The listing builds one solid part. Answer for the finished solid, in the listing's coordinates (mm). A direction names the side the tool comes from. Coordinates: 2 decimals unless noted, no trailing zeros. Order: outer loops, then holes, each group sorted by start corner. A loop starts at its lowest first (then second) coordinate and runs counter-clockwise, first axis right, second up. Notation, with made-up numbers: (-35, 4) -> (19, 4) arc R22 ccw to (19, 25) -> close; hole circle Ø3 at (23.5, 88.25). An arc over 180 degrees is marked (long way). Write each question's results on one line, items separated by ' | '. Start each with the question number.
(1) The part is cut by section B-B, the plane x = 61.5. Give the vertices of the cut face in (y, z).
(2) Straight lines are drawn through the part: L1, parallel to X at y = 6.75, z = -51; L2, parallel to X at y = 14.5, z = -8.5; L3, parallel to Z at x = 65, y = 19.75. For each, find the intervals that lie inside material, in ascending order.
(3) The part is cut by section C-C, the plane y = 10. Give the vertices of the cut face in (x, z), then the cut area to 3 significant figures.
(4) The part is cut by section D-D, the plane x = 87.5. Give the vertices of the cut face in (y, z), then the cut area to 3 significant figures.
(5) The part is cut by section A-A, the plane y = 21.5. Give the vertices of the cut face in (x, z), then the cut area to 3 significant figures.
(6) Determine the mould class of faces 4 (the face through (100, 12, -49)), 5 (the face through (50, 25, -10)), 6 (the face through (72, 14, -10)) for opening direction X: +X half, -X half, draft (parallel to the pull), parting line (faces both ways), or undercut.
(7) Given pin 1 (1.9 mm diameter, centred on x = 82, z = -57, fed in from +Y); pin 2 (3 mm diameter, centred on x = 70.5, z = -5.5, fed in from +Y); pin 3 (4 mm diameter, centred on x = 35, z = -68, fed in from +Y), each flat-ended and moving along its own axis, determine where each tip first touches the part or whether it passes through.
(8) A tool of negligible diameter and unlimited length cuts with its end or side. For faces 1 (the face through (86, 2, -72)), 2 (the face through (49, 18, -2.4)), 3 (the face through (49, 12, -100)), from which of +Z, -Z, +X, -X, +Y, -Y can it reach the whole face along a straight path? Write none if from no direction.
```python
from build123d import *

# Parameters (mm, degrees)
CROQUIS1_W              = 100
CROQUIS1_H              = 100
PLACABASE_DEPTH         = 3
CROQUIS2_W              = 100
CROQUIS2_H              = 100
CROQUIS2_W_2            = 95.2
CROQUIS2_H_2            = 95.2
PAREDES_DEPTH           = 21
CROQUIS4_W              = 26.4
CROQUIS4_H              = 10.4
ALOJAMIENTOSMOTOR_DEPTH = 12.4
CROQUIS6_W              = 2.4
CROQUIS6_H              = 95.2
NERVIOSRIGIDEZ_DEPTH    = 9
CROQUIS7_W              = 95.2
CROQUIS7_H              = 6
BLOQUECUNA_DEPTH        = 10
CROQUIS8_W              = 44
CROQUIS8_H              = 4
TORRESENSORES_DEPTH     = 22


with BuildPart() as part:
    # Croquis1 → PlacaBase (new body)
    with BuildSketch(Plane(origin=(0, 0, 0), x_dir=(1, 0, 0), z_dir=(0, 1, 0))):
        with Locations((50, 50)):
            Rectangle(CROQUIS1_W, CROQUIS1_H)
    extrude(amount=PLACABASE_DEPTH)

    # Croquis2 → Paredes (add)
    with BuildSketch(Plane(origin=(0, 3, 0), x_dir=(1, 0, 0), z_dir=(0, 1, 0))):
        with Locations((50, 50)):
            Rectangle(CROQUIS2_W, CROQUIS2_H)
        with Locations((50, 50)):
            Rectangle(CROQUIS2_W_2, CROQUIS2_H_2, mode=Mode.SUBTRACT)
    extrude(amount=PAREDES_DEPTH)

    # Croquis4 → AlojamientosMotor (cut)
    with BuildSketch(Plane(origin=(0, 7.3, 0), x_dir=(1, 0, 0), z_dir=(0, 1, 0))):
        with Locations((27.2, 72)):
            Rectangle(CROQUIS4_W, CROQUIS4_H)
        with Locations((72.8, 72)):
            Rectangle(CROQUIS4_W, CROQUIS4_H)
    extrude(amount=-ALOJAMIENTOSMOTOR_DEPTH, mode=Mode.SUBTRACT)

    # Croquis6 → NerviosRigidez (add)
    with BuildSketch(Plane(origin=(0, 3, 0), x_dir=(1, 0, 0), z_dir=(0, 1, 0))):
        with Locations((18.2, 50)):
            Rectangle(CROQUIS6_W, CROQUIS6_H)
        with Locations((81.8, 50)):
            Rectangle(CROQUIS6_W, CROQUIS6_H)
    extrude(amount=NERVIOSRIGIDEZ_DEPTH)

    # Croquis7 → BloqueCuna (add)
    with BuildSketch(Plane(origin=(0, 3, 0), x_dir=(1, 0, 0), z_dir=(0, 1, 0))):
        with Locations((50, 5.4)):
            Rectangle(CROQUIS7_W, CROQUIS7_H)
    extrude(amount=BLOQUECUNA_DEPTH)

    # Croquis8 → TorreSensores (add)
    with BuildSketch(Plane(origin=(0, 3, 0), x_dir=(1, 0, 0), z_dir=(0, 1, 0))):
        with Locations((50, 10.4)):
            Rectangle(CROQUIS8_W, CROQUIS8_H)
    extrude(amount=TORRESENSORES_DEPTH)


solid = part.part
```
Established:
1) outline: (0, -100) -> (24, -100) -> (24, -97.6) -> (3, -97.6) -> (3, -77.2) -> (0, -77.2) -> close; (0, -66.8) -> (3, -66.8) -> (3, -12.4) -> (25, -12.4) -> (25, -8.4) -> (13, -8.4) -> (13, -2.4) -> (24, -2.4) -> (24, 0) -> (0, 0) -> close
2) L1: x = 0 to 2.4, 17 to 19.4, 80.6 to 83, 97.6 to 100 | L2: x = 0 to 2.4, 28 to 72, 97.6 to 100 | L3: z = -100 to -97.6, -12.4 to -8.4, -2.4 to 0
3) outline: (0, -100) -> (100, -100) -> (100, 0) -> (0, 0) -> close; hole (2.4, -97.6) -> (17, -97.6) -> (17, -8.4) -> (2.4, -8.4) -> close; hole (19.4, -97.6) -> (80.6, -97.6) -> (80.6, -8.4) -> (72, -8.4) -> (72, -12.4) -> (28, -12.4) -> (28, -8.4) -> (19.4, -8.4) -> close; hole (83, -97.6) -> (97.6, -97.6) -> (97.6, -8.4) -> (83, -8.4) -> close | area: 2,110 mm^2
4) outline: (0, -100) -> (24, -100) -> (24, -97.6) -> (3, -97.6) -> (3, -8.4) -> (13, -8.4) -> (13, -2.4) -> (24, -2.4) -> (24, 0) -> (0, 0) -> close | area: 461 mm^2
5) outline: (0, -100) -> (100, -100) -> (100, 0) -> (0, 0) -> close; (28, -12.4) -> (72, -12.4) -> (72, -8.4) -> (28, -8.4) -> close; hole (2.4, -97.6) -> (97.6, -97.6) -> (97.6, -2.4) -> (2.4, -2.4) -> close | area: 1,110 mm^2
6) face 4: +X half | face 5: draft | face 6: undercut
7) pin 1: stops at y = 12 | pin 2: stops at y = 13 | pin 3: stops at y = 3
8) face 1: +Y, -Y | face 2: +Y | face 3: -Z, +X, -X, +Y, -Y
